from build123d import *

# Parameters (mm, degrees)
BOSS_EXTRUDE1_DEPTH   = 6
SKETCH2_W             = 6
SKETCH2_H             = 25
BOSS_EXTRUDE2_DEPTH   = 6
LPATTERN1_START       = 25
LPATTERN1_OUTLINE_W   = 6
LPATTERN1_OUTLINE_H   = 6
LPATTERN1_DEPTH       = 25
LPATTERN1_START_2     = 75
LPATTERN1_2_OUTLINE_W = 6
LPATTERN1_2_OUTLINE_H = 6
LPATTERN1_2_DEPTH     = 25
LPATTERN1_START_3     = 125
LPATTERN1_3_OUTLINE_W = 6
LPATTERN1_3_OUTLINE_H = 6
LPATTERN1_3_DEPTH     = 25
SKETCH5_R             = 4
CUT_EXTRUDE1_DEPTH    = 236.153141591


# Read off the part's stored shape, not the designer's step: LPattern1
with BuildPart() as part:
    # Sketch1 → Boss-Extrude1 (new body)
    with BuildSketch(Plane.XY):
        with BuildLine():
            Line((-150, 150), (-175, 150))
            Line((-175, 150), (-175, 0))
            Line((-175, 0), (0, 0))
            Line((0, 0), (0, 150))
            Line((0, 150), (-25, 150))
            Line((-25, 150), (-25, 110))
            ThreePointArc((-25, 110), (-32.083192968, 81.099697262), (-51.727279947, 58.75))
            ThreePointArc((-51.727279947, 58.75), (-87.5, 32.5), (-123.272720053, 58.75))
            ThreePointArc((-123.272720053, 58.75), (-142.916807032, 81.099697262), (-150, 110))
            Line((-150, 110), (-150, 150))
        make_face()
    extrude(amount=BOSS_EXTRUDE1_DEPTH)

    # Sketch2 → Boss-Extrude2 (add)
    with BuildSketch(Plane.XY.offset(6)):
        with Locations((-178, 137.5)):
            Rectangle(SKETCH2_W, SKETCH2_H)
    extrude(amount=-BOSS_EXTRUDE2_DEPTH)

    # LPattern1 outline → LPattern1 (add)
    with BuildSketch(Plane(origin=(0, 0, 0), x_dir=(1, 0, 0), z_dir=(0, 1, 0)).offset(LPATTERN1_START)):
        with Locations((-178, -3)):
            Rectangle(LPATTERN1_OUTLINE_W, LPATTERN1_OUTLINE_H)
        with Locations((3, -3)):
            Rectangle(LPATTERN1_OUTLINE_W, LPATTERN1_OUTLINE_H)
    extrude(amount=LPATTERN1_DEPTH)

    # LPattern1 2 outline → LPattern1 2 (add)
    with BuildSketch(Plane(origin=(0, 0, 0), x_dir=(1, 0, 0), z_dir=(0, 1, 0)).offset(LPATTERN1_START_2)):
        with Locations((-178, -3)):
            Rectangle(LPATTERN1_2_OUTLINE_W, LPATTERN1_2_OUTLINE_H)
        with Locations((3, -3)):
            Rectangle(LPATTERN1_2_OUTLINE_W, LPATTERN1_2_OUTLINE_H)
    extrude(amount=LPATTERN1_2_DEPTH)

    # LPattern1 3 outline → LPattern1 3 (add)
    with BuildSketch(Plane(origin=(0, 0, 0), x_dir=(1, 0, 0), z_dir=(0, 1, 0)).offset(LPATTERN1_START_3)):
        with Locations((3, -3)):
            Rectangle(LPATTERN1_3_OUTLINE_W, LPATTERN1_3_OUTLINE_H)
    extrude(amount=LPATTERN1_3_DEPTH)

    # Sketch5 → Cut-Extrude1 (cut, through all)
    with BuildSketch(Plane.XY.offset(6)):
        with Locations((-63.5, 25)):
            Circle(SKETCH5_R)
    extrude(amount=-CUT_EXTRUDE1_DEPTH, mode=Mode.SUBTRACT)


solid = part.part
Work out the finished part from the listing and answer in its coordinate system (mm). A direction names the side the tool comes from. Give positions to 0.01 mm unless a question says otherwise; leave off trailing zeros. Order: outer loops, then holes, each group sorted by start corner. A loop starts at its lowest first (then second) coordinate and runs counter-clockwise, first axis right, second up. Notation, with made-up numbers: M -36.75,-21.75 L 14.25,-21.75 A17 cw 14.25,-14.75 Z; hole C -12,43 d8. An arc over 180 degrees is marked long. Return JSON: item names as keys, results as strings.
Q1. Find section C-C, the plane x = -63.5. Write down the section's boundary in (y, z).
Answer below:
{"outline": "M 0,0 L 21,0 L 21,6 L 0,6 Z; M 29,0 L 41.19,0 L 41.19,6 L 29,6 Z"}
Q2. Find the intervals of material crossed by line 1 along X through (y, z) = (120, 2.7); line 2 along X through (y, z) = (132.5, 2.1); line 3 along X through (y, z) = (11, 1.15), in increasing order. Write a range as [from, to].
Answer below:
{"line 1": "x = [-175, -150], [-25, 0]", "line 2": "x = [-181, -150], [-25, 6]", "line 3": "x = [-175, 0]"}
Q3. Find section B-B, the plane y = 72. Write down the section's boundary in (x, z), and give its area (3 significant figures).
Answer below:
{"outline": "M -175,0 L -137.12,0 L -137.12,6 L -175,6 Z; M -37.88,0 L 0,0 L 0,6 L -37.88,6 Z", "area": "455 mm^2"}
Q4. The mould has two halves that part along X. Classify faces 5 (the face through (-86.835, 32.506, 2.958)), 6 (the face through (-175, 13, 3)), 7 (the face through (3, 125, 3)), 8 (the face through (-142.721, 80.727, 2.958)): pulls with the +X half, pulls with the -X half, needs draft (parallel to the pull), parting line crosses it, or undercut.
Answer below:
{"face 5": "undercut", "face 6": "pulls with the -X half", "face 7": "needs draft", "face 8": "undercut"}
Q5. Find section D-D, the plane x = -146. Write down the section's boundary in (y, z), and give its area (3 significant figures).
Answer below:
{"outline": "M 0,0 L 88,0 L 88,6 L 0,6 Z", "area": "528 mm^2"}
Q6. Each of these flat-tipped pins is pushed along its axis until it touches: pin 1 (3 mm diameter, centred on y = 18.5, z = 4, fed in from -X); pin 2 (1.8 mm diameter, centred on y = 108.5, z = 1.5, fed in from +X); pin 3 (1.8 mm diameter, centred on x = -178.5, z = 3.5, fed in from -Y). Where does it stop, or does it pass through?
Answer below:
{"pin 1": "stops at x = -175", "pin 2": "stops at x = 0", "pin 3": "stops at y = 25"}
Q7. Which of the six approach directions +Z, -Z, +X, -X, +Y, -Y give full straight-line access (tool end or side, diameter ignored) to faces 1 (the face through (-25, 130, 3)), 2 (the face through (-178, 25, 3)), 3 (the face through (0, 12, 3)), 4 (the face through (-175, 113, 3))?
Answer below:
{"face 1": "+Z, -Z, +Y", "face 2": "+Z, -Z, -X, -Y", "face 3": "+Z, -Z, +X, -Y", "face 4": "+Z, -Z, -X"}
